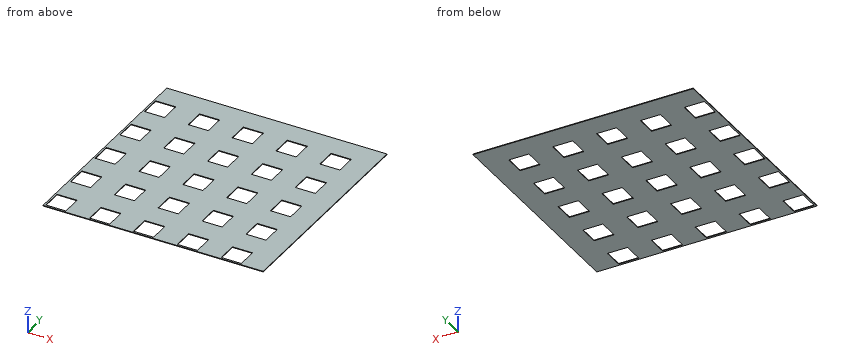
from build123d import *

# Parameters (mm, degrees)
F0_W     = 100
F0_H     = 100
F0_W_2   = 9.12
F0_H_2   = 9.12
F1_DEPTH = 0.3


with BuildPart() as f1:
    # F0 (on Top) → F1 (new body)
    with BuildSketch(Plane.XY):
        with Locations((50, 50)):
            Rectangle(F0_W, F0_H)
        with Locations((5.36, 5.36)):
            Rectangle(F0_W_2, F0_H_2, mode=Mode.SUBTRACT)
        with Locations((25.28, 5.36)):
            Rectangle(F0_W_2, F0_H_2, mode=Mode.SUBTRACT)
        with Locations((45.2, 5.36)):
            Rectangle(F0_W_2, F0_H_2, mode=Mode.SUBTRACT)
        with Locations((5.36, 25.28)):
            Rectangle(F0_W_2, F0_H_2, mode=Mode.SUBTRACT)
        with Locations((5.36, 45.2)):
            Rectangle(F0_W_2, F0_H_2, mode=Mode.SUBTRACT)
        with Locations((25.28, 25.28)):
            Rectangle(F0_W_2, F0_H_2, mode=Mode.SUBTRACT)
        with Locations((45.2, 25.28)):
            Rectangle(F0_W_2, F0_H_2, mode=Mode.SUBTRACT)
        with Locations((25.28, 45.2)):
            Rectangle(F0_W_2, F0_H_2, mode=Mode.SUBTRACT)
        with Locations((45.2, 45.2)):
            Rectangle(F0_W_2, F0_H_2, mode=Mode.SUBTRACT)
        with Locations((65.12, 5.36)):
            Rectangle(F0_W_2, F0_H_2, mode=Mode.SUBTRACT)
        with Locations((85.04, 5.36)):
            Rectangle(F0_W_2, F0_H_2, mode=Mode.SUBTRACT)
        with Locations((65.12, 25.28)):
            Rectangle(F0_W_2, F0_H_2, mode=Mode.SUBTRACT)
        with Locations((65.12, 45.2)):
            Rectangle(F0_W_2, F0_H_2, mode=Mode.SUBTRACT)
        with Locations((85.04, 25.28)):
            Rectangle(F0_W_2, F0_H_2, mode=Mode.SUBTRACT)
        with Locations((85.04, 45.2)):
            Rectangle(F0_W_2, F0_H_2, mode=Mode.SUBTRACT)
        with Locations((5.36, 65.12)):
            Rectangle(F0_W_2, F0_H_2, mode=Mode.SUBTRACT)
        with Locations((25.28, 65.12)):
            Rectangle(F0_W_2, F0_H_2, mode=Mode.SUBTRACT)
        with Locations((45.2, 65.12)):
            Rectangle(F0_W_2, F0_H_2, mode=Mode.SUBTRACT)
        with Locations((5.36, 85.04)):
            Rectangle(F0_W_2, F0_H_2, mode=Mode.SUBTRACT)
        with Locations((25.28, 85.04)):
            Rectangle(F0_W_2, F0_H_2, mode=Mode.SUBTRACT)
        with Locations((45.2, 85.04)):
            Rectangle(F0_W_2, F0_H_2, mode=Mode.SUBTRACT)
        with Locations((65.12, 65.12)):
            Rectangle(F0_W_2, F0_H_2, mode=Mode.SUBTRACT)
        with Locations((85.04, 65.12)):
            Rectangle(F0_W_2, F0_H_2, mode=Mode.SUBTRACT)
        with Locations((65.12, 85.04)):
            Rectangle(F0_W_2, F0_H_2, mode=Mode.SUBTRACT)
        with Locations((85.04, 85.04)):
            Rectangle(F0_W_2, F0_H_2, mode=Mode.SUBTRACT)
    extrude(amount=F1_DEPTH)


solid = f1.part
Can you work these out from the model? Positions are in its coordinate system, mm. Round coordinates to 2 decimals unless told otherwise and drop trailing zeros. Write each loop counter-clockwise with the first axis right and the second up, starting at its lowest first coordinate (ties: lowest second). Pieces come first, ordered by that corner, then holes. Notation, with made-up numbers: (-18.5, 25.25) -> (0.5, 25.25) arc R14 cw to (0.5, 44.25) -> close; hole circle Ø6 at (9.5, -24.75). An arc over 180 degrees is marked (long way). Use one line per item in the form item = value. Start each with the question number.
Q1. Imagine slicing it at A-A (y = 82.5). Please give me the cut outline in (x, z), then the cut area to 3 significant figures.
Q2. Imagine slicing it at C-C (z = 0.1). Count the separate pieces of the cut face and the enclosed holes in it, then the cut area to 3 significant figures.
Q3. If I drill on probe 1 along X at (y, z) = (22.5, 0.1), over which ranges is the centre line in solid material (lowest first)? Write a range as [from, to].
Worked out:
q1.outline = (0, 0) -> (0.8, 0) -> (0.8, 0.3) -> (0, 0.3) -> close; (9.92, 0) -> (20.72, 0) -> (20.72, 0.3) -> (9.92, 0.3) -> close; (29.84, 0) -> (40.64, 0) -> (40.64, 0.3) -> (29.84, 0.3) -> close; (49.76, 0) -> (60.56, 0) -> (60.56, 0.3) -> (49.76, 0.3) -> close; (69.68, 0) -> (80.48, 0) -> (80.48, 0.3) -> (69.68, 0.3) -> close; (89.6, 0) -> (100, 0) -> (100, 0.3) -> (89.6, 0.3) -> close
q1.area = 16.3 mm^2
q2.separate_pieces = 1
q2.enclosed_holes = 25
q2.area = 7,920 mm^2
q3.probe_1 = [0, 0.8], [9.92, 20.72], [29.84, 40.64], [49.76, 60.56], [69.68, 80.48], [89.6, 100]
